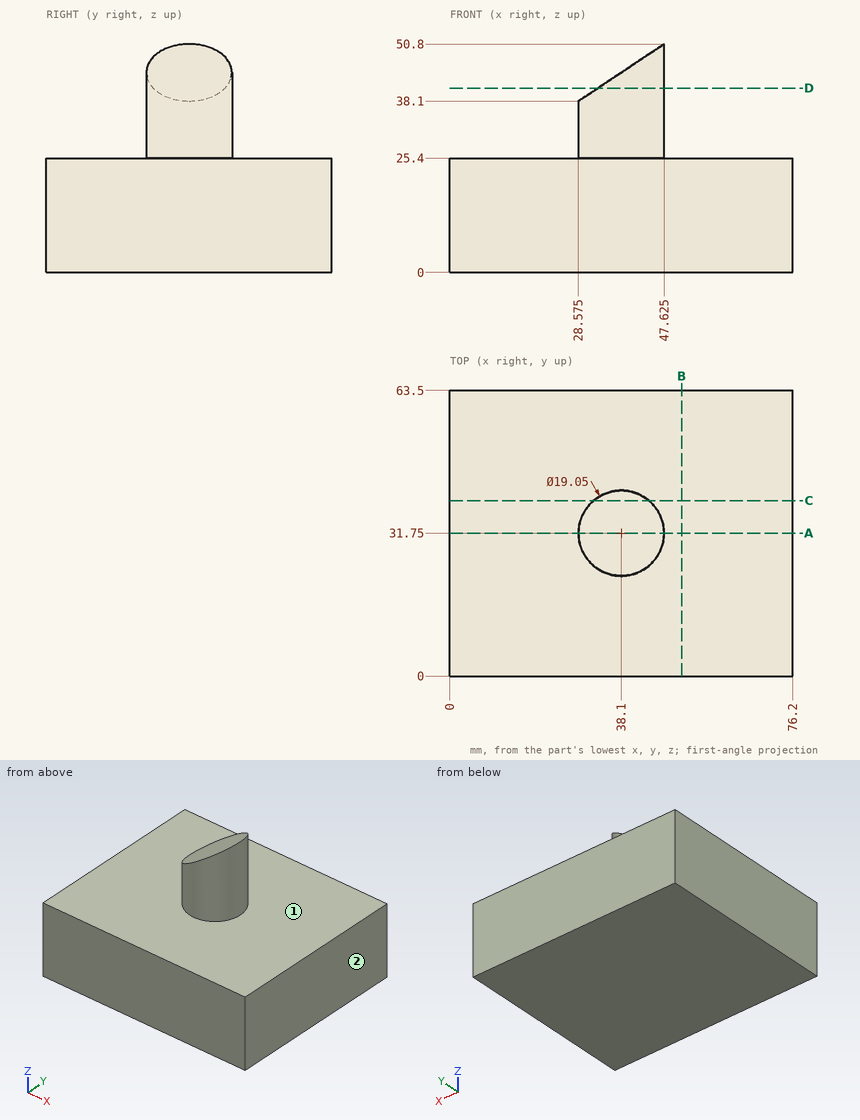
Drawing for the job (mm, zero at the part's lowest x, y, z). A direction names the side the tool comes from. Round coordinates to 2 decimals unless told otherwise and drop trailing zeros. Loops run counter-clockwise (first coordinate to the right, second up) from the corner with the lowest first, then second, coordinate; pieces in that order, holes last. Notation, with made-up numbers: (12.5, 2) -> (67.5, 2) arc R22 cw to (67.5, 29) -> close; hole circle Ø1 at (10, -34.5). An arc over 180 degrees is marked (long way). Answer in a Markdown table with one row per item.
Item 1: Saw through at B-B (x = 51.5). Write the cut outline in (y, z), and give its area (3 significant figures).
Answers below:
| item | result |
|---|---|
| outline | (0, 0) -> (63.5, 0) -> (63.5, 25.4) -> (0, 25.4) -> close |
| area | 1,610 mm² |
Item 2: Drill centre lines: L1, parallel to Z at x = 39.5, y = 8.5; L2, parallel to Z at x = 43, y = 38.5; L3, parallel to X at y = 29, z = 27. Where is each one in solid material? Low to high. Write a range as [from, to].
Answers below:
| item | result |
|---|---|
| L1 | z = [0, 25.4] |
| L2 | z = [0, 47.72] |
| L3 | x = [28.98, 47.22] |
Item 3: Saw through at D-D (z = 41). Write the cut outline in (x, y) (3 decimals).
Answers below:
| item | result |
|---|---|
| outline | (32.925, 23.753) arc R9.525 ccw (long way) to (32.925, 39.747) -> close |
Item 4: Saw through at A-A (y = 31.75). Write the cut outline in (x, z) (3 decimals), and give its area (3 significant figures).
Answers below:
| item | result |
|---|---|
| outline | (0, 0) -> (76.2, 0) -> (76.2, 25.4) -> (47.625, 25.4) -> (47.625, 50.8) -> (28.575, 38.1) -> (28.575, 25.4) -> (0, 25.4) -> close |
| area | 2,300 mm² |
Item 5: Saw through at C-C (y = 39). Write the cut outline in (x, z).
Answers below:
| item | result |
|---|---|
| outline | (0, 0) -> (76.2, 0) -> (76.2, 25.4) -> (44.28, 25.4) -> (44.28, 48.57) -> (31.92, 40.33) -> (31.92, 25.4) -> (0, 25.4) -> close |
Item 6: Which spindle directions (+Z, -Z, +X, -X, +Y, -Y) get a long thin tool onto all of the face, cutting with end or side? Do the marked faces 1 and 2. Say none if no direction does.
Answers below:
| item | result |
|---|---|
| face 1 | +Z |
| face 2 | +Z, -Z, +X, +Y, -Y |
Item 7: Pin check, flat tips, straight feed: pin 1 (12 mm diameter, centred on y = 16, z = 36.5, fed in from +X); pin 2 (5 mm diameter, centred on x = 68.5, y = 23.5, fed in from +Z). Stop position of each tip, or through.
Answers below:
| item | result |
|---|---|
| pin 1 | passes through |
| pin 2 | stops at z = 25.4 |
